Job drawing, mm, ordinate dimensions from the low corner. One solid piece. A direction names the side the tool comes from. Round coordinates to 2 decimals unless told otherwise and drop trailing zeros. Order: outer loops, then holes, each group sorted by start corner. A loop starts at its lowest first (then second) coordinate and runs counter-clockwise, first axis right, second up. Notation, with made-up numbers: (15, 62) -> (32, 62) arc R17 ccw to (32, 70) -> close; hole circle Ø6 at (51, 59). An arc over 180 degrees is marked (long way). Write item = value, one per line.
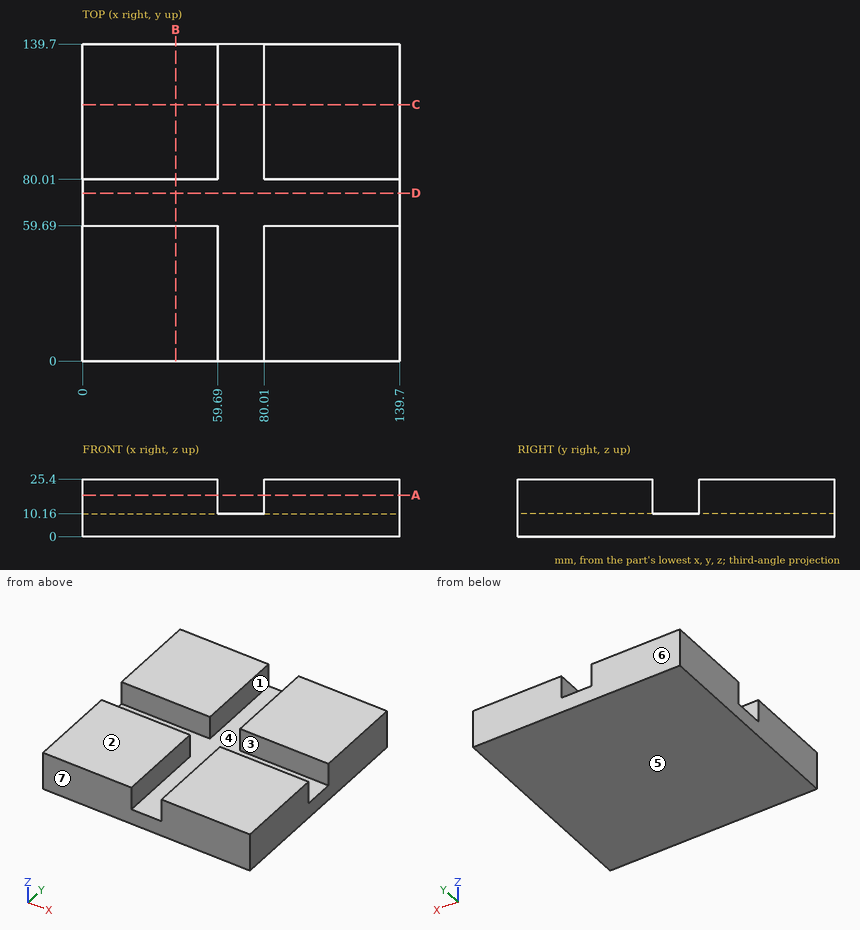
Q1. Which spindle directions (+Z, -Z, +X, -X, +Y, -Y) get a long thin tool onto all of the face, cutting with end or side? Do the marked faces 1, 2 and 3. Say none if no direction does.
Check values:
face_1 = +Z, +Y, -Y
face_2 = +Z, +X, -X, +Y, -Y
face_3 = +Z, +X, -X
Q2. Flat gauge pin, fed straight in: pin 1 (6 mm diameter, centred on x = 74.5, z = 21, fed in from -Y). Where does the tip first touch, or does it go through?
Check values:
pin_1 = through
Q3. Cut at A-A, the plane z = 18.25. List the corners of the cut face in (x, y).
Check values:
outline = (0, 0) -> (59.69, 0) -> (59.69, 59.69) -> (0, 59.69) -> close; (0, 80.01) -> (59.69, 80.01) -> (59.69, 139.7) -> (0, 139.7) -> close; (80.01, 0) -> (139.7, 0) -> (139.7, 59.69) -> (80.01, 59.69) -> close; (80.01, 80.01) -> (139.7, 80.01) -> (139.7, 139.7) -> (80.01, 139.7) -> close
Q4. Cut at D-D, the plane y = 74. List the corners of the cut face in (x, z), and give its area (3 significant figures).
Check values:
outline = (0, 0) -> (139.7, 0) -> (139.7, 10.16) -> (0, 10.16) -> close
area = 1,420 mm²
Q5. Cut at B-B, the plane x = 41. List the corners of the cut face in (y, z).
Check values:
outline = (0, 0) -> (139.7, 0) -> (139.7, 25.4) -> (80.01, 25.4) -> (80.01, 10.16) -> (59.69, 10.16) -> (59.69, 25.4) -> (0, 25.4) -> close
Q6. Mould opens along Y. For the marked faces 4, 5, 6 and 7 say: released by +Y, released by -Y, zero draft, split by the parting line, or undercut.
Check values:
face_4 = undercut
face_5 = zero draft
face_6 = released by +Y
face_7 = released by -Y
Q7. Probe probe 1 along X at (y, z) = (110, 19.5); probe 2 along Z at (x, y) = (76, 104.5). List the from-to ranges inside material, lowest first.
Check values:
probe_1 = 0 to 59.69, 80.01 to 139.7
probe_2 = 0 to 10.16
